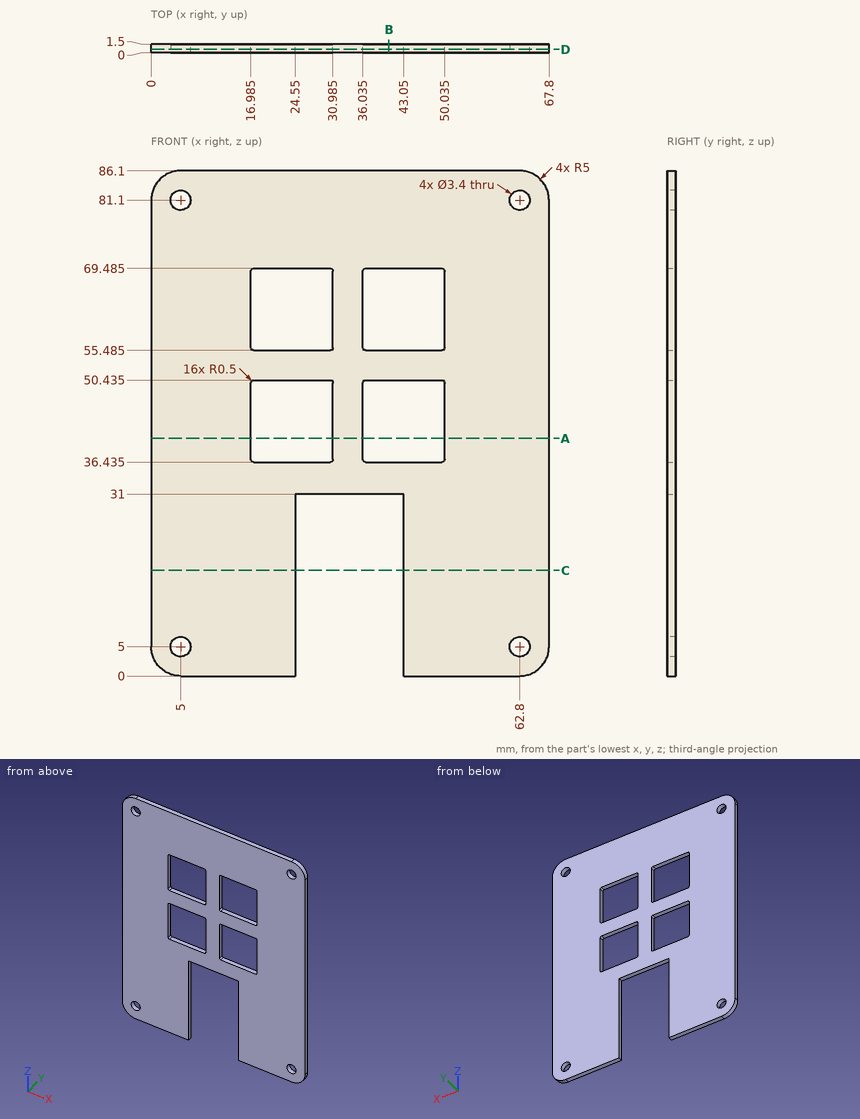
The figure shows three views and two pictorial views of one solid part (mm, origin at its lowest corner). Answer the questions. Coordinates: 2 decimals unless noted, no trailing zeros. Order: outer loops, then holes, each group sorted by start corner. A loop starts at its lowest first (then second) coordinate and runs counter-clockwise, first axis right, second up. Notation, with made-up numbers: (14, 40) - (67, 40) arc R8 cw to (67, 54) - close; hole circle Ø11 at (22, -9). An arc over 180 degrees is marked (long way). Answer as a JSON object with one key per item and string values.
1. Each of these flat-tipped pins is pushed along its axis until it touches: P1, Ø0.8, axis at x = 26, y = 1, coming from the -Z side; P2, Ø2.5, axis at x = 5, z = 81.1, coming from the -Y side. Where does it stop, or does it pass through?
Output values:
{"P1": "stops at z = 31", "P2": "passes through"}
2. Find section A-A on z = 40.5. Determine the outline of the cut face in (x, y) (3 decimals).
Output values:
{"outline": "(0, 0) - (16.985, 0) - (16.985, 1.5) - (0, 1.5) - close; (30.985, 0) - (36.035, 0) - (36.035, 1.5) - (30.985, 1.5) - close; (50.035, 0) - (67.8, 0) - (67.8, 1.5) - (50.035, 1.5) - close"}
3. Find section C-C on z = 18. Determine the outline of the cut face in (x, y).
Output values:
{"outline": "(0, 0) - (24.55, 0) - (24.55, 1.5) - (0, 1.5) - close; (43.05, 0) - (67.8, 0) - (67.8, 1.5) - (43.05, 1.5) - close"}
4. Find section B-B on x = 40.5. Determine the outline of the cut face in (y, z) (3 decimals), plus the area to 4 significant figures.
Output values:
{"outline": "(0, 31) - (1.5, 31) - (1.5, 36.435) - (0, 36.435) - close; (0, 50.435) - (1.5, 50.435) - (1.5, 55.485) - (0, 55.485) - close; (0, 69.485) - (1.5, 69.485) - (1.5, 86.1) - (0, 86.1) - close", "area": "40.65 mm²"}
5. Find section D-D on y = 0.6. Count the separate pieces of the cut face and the enclosed holes in it, plus the area to 3 significant figures.
Output values:
{"separate pieces": "1", "enclosed holes": "8", "area": "4,420 mm²"}
6. Consider line 1 (Z direction, x = 5, y = 0.55); line 2 (Z direction, x = 25.5, y = 1.1) (3 decimals); line 3 (X direction, y = 0.55, z = 81.1). Determine where each line is inside the solid, lowest interval first.
Output values:
{"line 1": "z = 0 to 3.3, 6.7 to 79.4, 82.8 to 86.1", "line 2": "z = 31 to 36.435, 50.435 to 55.485, 69.485 to 86.1", "line 3": "x = 0 to 3.3, 6.7 to 61.1, 64.5 to 67.8"}
